Autodesk Inventor part; units mm, degrees
ref_plane "YZ Plane" through (0, 0, 0) normal (1, 0, 0) x (0, 1, 0)
ref_plane "XZ Plane" through (0, 0, 0) normal (0, 1, 0) x (-1, 0, 0)
ref_plane "XY Plane" through (0, 0, 0) normal (0, 0, 1) x (1, 0, 0)
sketch "Sketch1" plane through (0, 0, 0) normal (0, 0, 1) x (1, 0, 0)
  line L0 (-18.9826, -15.7) -> (4.0174, -15.7)
  line L1 (11.5, 10) -> (11.5, -10)
  line L2 (11.5, -10) -> (-11.5, -10)
  line L3 (-11.5, -10) -> (-11.5, 10)
  line L4 (-11.5, 10) -> (11.5, 10)
  line L5 (-18.9826, -15.7) -> (-18.9826, -14)
  line L6 (-18.9826, -15.7) -> (-18.9826, -18.2)
  line L7 (-18.9826, -18.2) -> (11.5, -18.2)
  line L8 (11.5, -18.2) -> (11.5, 10)
  line L9 (11.5, 10) -> (-18.9826, 10)
  line L10 (-18.9826, 10) -> (-18.9826, -18.2)
  point P0 (0, 0)
  dimension "d0" = 2.5
extrude "Extrusion1" add sketch "Sketch1" along normal blind 2.5
sketch "Sketch2" plane through (0, 0, 0) normal (0, 0, -1) x (-1, 0, 0)
  line L0 (18.9826, 10) -> (18.9826, -18.2)
  line L1 (-11.5, -18.2) -> (-11.5, 10)
  line L2 (18.9826, -18.2) -> (-11.5, -18.2)
  line L3 (-11.5, -18.2) -> (-11.5, -15.7)
  line L4 (-11.5, -15.7) -> (18.9826, -15.7)
  line L5 (18.9826, -15.7) -> (18.9826, -18.2)
  point P0 (0, 0)
  dimension "d3" = 2.5
extrude "Extrusion2" add sketch "Sketch2" along normal blind 40
sketch "Sketch4" plane through (-18.9826, -15.7, 0) normal (0, 1, 0) x (1, 0, 0)
  line L0 (23, 13.2181) -> (23, 36.2181)
  line L1 (23, 36.2181) -> (0, 36.2181)
  line L2 (0, 36.2181) -> (0, 13.2181)
  line L3 (0, 13.2181) -> (23, 13.2181)
  circle A0 centre (20.5, 15.7181) radius 1.5
  circle A1 centre (20.5, 33.7181) radius 1.5
  circle A2 centre (2.5, 33.7181) radius 1.5
  circle A3 centre (2.5, 15.7181) radius 1.5
  point P0 (18.9826, 0)
extrude "Extrusion3" cut sketch "Sketch4" against normal blind 40 contours A0 | A1 | A2 | A3
sketch "Sketch5" plane through (0, 0, 0) normal (0, 0, -1) x (-1, 0, 0)
  line L0 (9.8803, 8.3507) -> (9.8803, -8.3507)
  line L1 (9.8803, -8.3507) -> (5.0848, -8.3507)
  line L2 (5.0848, -8.3507) -> (5.0848, 8.3507)
  line L3 (5.0848, 8.3507) -> (9.8803, 8.3507)
  line L4 (-11.5, -10) -> (11.5, -10)
  line L5 (11.5, -10) -> (11.5, 10)
  line L6 (11.5, 10) -> (-11.5, 10)
  line L7 (-11.5, 10) -> (-11.5, -10)
  circle A0 centre (-9, -7) radius 1.5
  circle A1 centre (-9, 7) radius 1.5
  point P0 (0, 0)
extrude "Extrusion4" cut sketch "Sketch5" against normal blind 40 contours A0 | A1
ref_plane "Work Plane1" through (-2.2662, 39.9957, 12.7819) normal (0, 0, 1) x (-0.8579373, 0.5137544, 0)
sketch "Sketch6" plane through (-2.2662, 39.9957, 12.7819) normal (0, 0, 1) x (-0.8579373, 0.5137544, 0)
  line L0 (18.5, 0) -> (18.5, 93.5988)
  line L1 (-1.5, 0) -> (-1.5, 93.5988)
  line L2 (21.5, 18.6957) -> (-3.5, 18.6957)
  line L3 (-4.5, 75.0357) -> (21.5, 75.0357)
  line L4 (-15.5567, 58.5163) -> (-41.7088, 42.8558)
  line L5 (-15.5567, 58.5163) -> (18.5, 58.5163)
  line L6 (-27.221, 18.662) -> (-1.0688, 34.3225)
  line L7 (-1.0688, 34.3225) -> (18.5, 34.3225)
  line L8 (-1.5, 34.0643) -> (-15.9879, 58.2581)
  line L9 (-1.0688, 34.3225) -> (-1.6546, 34.3225)
  point P0 (-22.4922, 33.1495)
extrude "Extrusion5" add sketch "Sketch6" along normal blind 2.5 contours L7 L9 L1 L5 L0 | L1 L9 L8 L4 L5
sketch "Sketch7" plane through (-2.2662, 39.9957, 15.2819) normal (0, 0, 1) x (0.8579373, -0.5137544, 0)
  line L0 (15.5567, -58.5163) -> (41.7088, -42.8558)
  line L1 (15.9879, -58.2581) -> (18.1327, -56.9738)
  line L2 (1.6546, -34.3225) -> (-18.5, -34.3225)
  line L3 (1.6546, -34.3225) -> (5.6436, -31.9338)
  line L4 (15.9879, -58.2581) -> (1.6546, -34.3225)
  line L5 (18.1327, -56.9738) -> (1.8582, -29.7964)
  point P0 (22.4922, -33.1495)
  point P1 (3.7995, -33.0381)
  dimension "d12" = 2.5
  dimension "d13" = 2.5
extrude "Extrusion6" add sketch "Sketch7" against normal up to surface (12.7819 mm away)
sketch "Sketch8" plane through (-18.9826, -18.2, -40) normal (0, -1, 0) x (1, 0, 0)
  line L0 (3.0026, 55.2819) -> (3.0026, 42.5)
  line L1 (30.4826, 0) -> (30.4826, 42.5)
  line L2 (3.0026, 55.2819) -> (30.4826, 42.5)
  line L3 (30.4826, 42.5) -> (3.0026, 42.5)
  point P0 (18.9826, 40)
extrude "Extrusion7" add sketch "Sketch8" against normal blind 3
ref_plane "Work Plane4" through (9, 0, 0) normal (0, 1, 0) x (0, 0, 1)
ref_plane "Work Plane2" through (9, -7, 0) normal (0, 1, 0) x (0, 0, 1)
ref_plane "Work Plane3" through (9, 7, 2.5) normal (0, 1, 0) x (0, 0, -1)
sketch "Sketch9" plane through (9, 0, 0) normal (0, 1, 0) x (0, 0, 1)
  line L0 (-40, 2.5) -> (2.5, 2.5)
  line L1 (15.2819, -24.98) -> (15.2819, -27.48)
  line L2 (2.5, 2.5) -> (15.2819, -24.98)
  line L3 (15.2819, -24.98) -> (2.5, -24.98)
  line L4 (2.5, -24.98) -> (15.2819, -24.98)
  line L5 (2.5, 2.5) -> (2.5, -27.9826)
  line L6 (2.5, -24.98) -> (2.5, 2.5)
  point P0 (0, -9)
extrude "Extrusion8" add sketch "Sketch9" along normal mid plane 3
sketch "Sketch10" plane through (-2.2662, 39.9957, 15.2819) normal (0, 0, 1) x (0.8579373, -0.5137544, 0)
  line L0 (-6.3751, 0) -> (-6.3751, -93.5988)
  line L1 (-10.4351, 0) -> (-10.4351, -93.5988)
  line L2 (-6.3751, -46.7994) -> (-10.4351, -46.7994)
  circle A0 centre (-8.4051, -46.7994) radius 1.5
  line L3 (1.6546, -34.3225) -> (-18.5, -34.3225)
  line L4 (-6.3751, -34.3225) -> (-6.3751, -46.7994)
  line L5 (-6.3751, -40.561) -> (-10.4351, -40.561)
  line L6 (-18.5, -58.5163) -> (15.5567, -58.5163)
  line L7 (-6.3751, -58.5163) -> (-6.3751, -46.7994)
  line L8 (-6.3751, -52.6579) -> (-10.4351, -52.6579)
  circle A1 centre (-8.4051, -52.6579) radius 1.5
  circle A2 centre (-8.4051, -40.561) radius 1.5
  point P0 (22.4922, -33.1495)
  dimension "d22" = 3
  dimension "d23" = 3
  dimension "d24" = 3
extrude "Extrusion9" cut sketch "Sketch10" against normal blind 3 contours A2 L5 | L5 A2 | A1 L8 | L8 A1
properties part number "counter_sensor_holders" material "PET Plastic"
Geometry: final body of the model. Coordinates: model frame, mm. A direction names the side the tool comes from. Give positions to 0.01 mm unless a question says otherwise; leave off trailing zeros. Order: outer loops, then holes, each group sorted by start corner. A loop starts at its lowest first (then second) coordinate and runs counter-clockwise, first axis right, second up. Notation, with made-up numbers: (-1, 39) -> (51, 39) arc R18 ccw to (51, 73) -> close; hole circle Ø2 at (10.25, 76.5). An arc over 180 degrees is marked (long way). Put each result on its own line as item: value.
Q1. Pin query (flat end, axial travel): pin 1 (9 mm diameter, centred on x = 1.5, z = -12, fed in from +Y); pin 2 (6.5 mm diameter, centred on x = -6, z = 10.5, fed in from +Y); pin 3 (8 mm diameter, centred on x = -18.5, y = 1.5, fed in from -Z). Return the tip coordinate at first contact, or that it passes through.
Here are the results:
pin 1: stops at y = -15.7
pin 2: stops at y = 1.5
pin 3: stops at z = 0
Q2. Section A-A, the plane y = -7. Return loops of the section in (x, z), then the cut area to 3 significant figures.
Here are the results:
outline: (-37.69, 12.78) -> (-18.48, 12.78) -> (-18.48, 2.5) -> (-18.98, 2.5) -> (-18.98, 0) -> (7.5, 0) -> (7.5, 2.5) -> (-15.98, 2.5) -> (-15.98, 15.28) -> (-37.69, 15.28) -> close; (10.5, 0) -> (11.5, 0) -> (11.5, 2.5) -> (10.5, 2.5) -> close
area: 149 mm^2
Q3. Reachability of faces 4 (the face through (-4, -15.7, -20)), 5 (the face through (-9, -15.2, 6)), 6 (the face through (-18.983, -17, -9)) from +Z, -Z, +X, -X, +Y, -Y: full face, straight path, thin tool, end or side. Return the list, or none.
Here are the results:
face 4: -Z, +X, -X, +Y
face 5: +Z, +X
face 6: -Z, -X, +Y, -Y
Q4. Material intervals for L1, parallel to Y at x = 9, z = 0.6; L2, parallel to Y at x = 5.5, z = -35; L3, parallel to Z at x = -35, y = 10, sorted ascending.
Here are the results:
L1: y = -18.2 to -8.5, -5.5 to 5.5, 8.5 to 10
L2: y = -18.2 to -15.7
L3: z = 12.78 to 15.28
Q5. Section B-B, the plane x = 9. Return loops of the section in (y, z), then the cut area to 3 significant figures.
Here are the results:
outline: (-18.2, -40) -> (-15.7, -40) -> (-15.7, 0) -> (-8.5, 0) -> (-8.5, 2.5) -> (-15.2, 2.5) -> (-15.2, 3.66) -> (-18.2, 3.66) -> close; (-5.5, 0) -> (5.5, 0) -> (5.5, 2.5) -> (1.5, 2.5) -> (1.5, 3.66) -> (-1.5, 3.66) -> (-1.5, 2.5) -> (-5.5, 2.5) -> close; (8.5, 0) -> (10, 0) -> (10, 2.5) -> (8.5, 2.5) -> close
area: 162 mm^2
Q6. Section D-D, the plane x = -14. Return loops of the section in (y, z), then the cut area to 3 significant figures.
Here are the results:
outline: (-18.2, -40) -> (-15.7, -40) -> (-15.7, 0) -> (10, 0) -> (10, 2.5) -> (1.5, 2.5) -> (1.5, 14.36) -> (-1.5, 14.36) -> (-1.5, 2.5) -> (-15.2, 2.5) -> (-15.2, 14.36) -> (-18.2, 14.36) -> close
area: 242 mm^2
Q7. Draft query along Y for faces 1 (the face through (-28.974, 10.186, 14.049)), 2 (the face through (11.5, -17, -9)), 3 (the face through (-33.387, -9.574, 14.014)). Return one class per face: released by +Y, released by -Y, zero draft, split by the parting line, or undercut.
Here are the results:
face 1: undercut
face 2: zero draft
face 3: released by -Y
Q8. Section C-C, the plane z = 7. Return loops of the section in (x, y).
Here are the results:
outline: (-18.48, -18.2) -> (-15.98, -18.2) -> (1.83, -18.2) -> (1.83, -15.2) -> (-15.98, -15.2) -> (-15.98, -1.5) -> (1.83, -1.5) -> (1.83, 1.5) -> (-15.98, 1.5) -> (-15.98, 9.7) -> (-18.48, 9.7) -> close
